Autodesk Inventor part; units mm, degrees
ref_plane "YZ Plane" through (0, 0, 0) normal (1, 0, 0) x (0, 1, 0)
ref_plane "XZ Plane" through (0, 0, 0) normal (0, 1, 0) x (-1, 0, 0)
ref_plane "XY Plane" through (0, 0, 0) normal (0, 0, 1) x (1, 0, 0)
sketch "スケッチ1" plane through (0, 0, 0) normal (0, 0, 1) x (1, 0, 0)
  circle A0 centre (0, 0) radius 6
  dimension "d0" = 12
extrude "押し出し1" add sketch "スケッチ1" along normal blind 1
sketch "スケッチ2" plane through (0, 0, 1) normal (0, 0, 1) x (1, 0, 0)
  circle A0 centre (0, 0) radius 4
  circle A1 centre (0, 0) radius 3
  dimension "d3" = 8
  dimension "d4" = 6
extrude "押し出し2" add sketch "スケッチ2" along normal blind 5 contours A0 | A1
sketch "スケッチ3" plane through (0, 0, 6) normal (0, 0, 1) x (1, 0, 0)
  circle A0 centre (0, 0) radius 4
  circle A1 centre (0, 0) radius 3
  dimension "d7" = 6
extrude "押し出し3" cut sketch "スケッチ3" against normal blind 6 contours A1
properties part number "フランジブッシュ　d6-D8-l5-h12" material "アセタール樹脂、黒"
Model file for the job. Use its own axes, mm. Give positions to 0.01 mm unless a question says otherwise; leave off trailing zeros. Loops run counter-clockwise (first coordinate to the right, second up) from the corner with the lowest first, then second, coordinate; pieces in that order, holes last. Notation, with made-up numbers: (-23, 88) - (2, 88) arc R20 cw to (2, 109) - close; hole circle Ø5 at (65, -6). An arc over 180 degrees is marked (long way). One line per item, written item: value. Start each with the question number.
1. Slice it at A-A (x = 0). List the corners of the cut face in (y, z).
2. Pin check, flat tips, straight feed: pin 1 (1 mm diameter, centred on x = 2, z = 5.5, fed in from -Y); pin 2 (1 mm diameter, centred on y = 0, z = 5, fed in from +X); pin 3 (2 mm diameter, centred on y = 4.5, z = 1, fed in from +X). Stop position of each tip, or through.
3. Slice it at D-D (x = -5). List the corners of the cut face in (y, z), plus the area to 3 significant figures.
4. Slice it at C-C (z = 4.95). List the corners of the cut face in (x, y).
5. Probe L1, parallel to Y at x = 0, z = 1.85; L2, parallel to Z at x = 2, y = -5; L3, parallel to Y at x = 2.5, z = 1.95. List the from-to ranges inside material, lowest first. Write a range as from..to.
6. Pull direction X, two halves, no side cores. Call faces 1 (the cylindrical face through (-3, 0, 3)), 2 (the cylindrical face through (-0.867, 3.905, 3.465)), 3 (the flat face through (-1.42, -3.92, 1)): pulls with the +X half, pulls with the -X half, needs draft (parallel to the pull), parting line crosses it, or undercut.
Solution:
1. outline: (-6, 0) - (-3, 0) - (-3, 6) - (-4, 6) - (-4, 1) - (-6, 1) - close; (3, 0) - (6, 0) - (6, 1) - (4, 1) - (4, 6) - (3, 6) - close
2. pin 1: stops at y = -3.71
2. pin 2: stops at x = 4
2. pin 3: stops at x = 4.87
3. outline: (-3.32, 0) - (3.32, 0) - (3.32, 1) - (-3.32, 1) - close
3. area: 6.63 mm^2
4. outline: circle Ø8 at (0, 0); hole circle Ø6 at (0, 0)
5. L1: y = -4..-3, 3..4
5. L2: z = 0..1
5. L3: y = -3.12..-1.66, 1.66..3.12
6. face 1: undercut
6. face 2: parting line crosses it
6. face 3: needs draft
